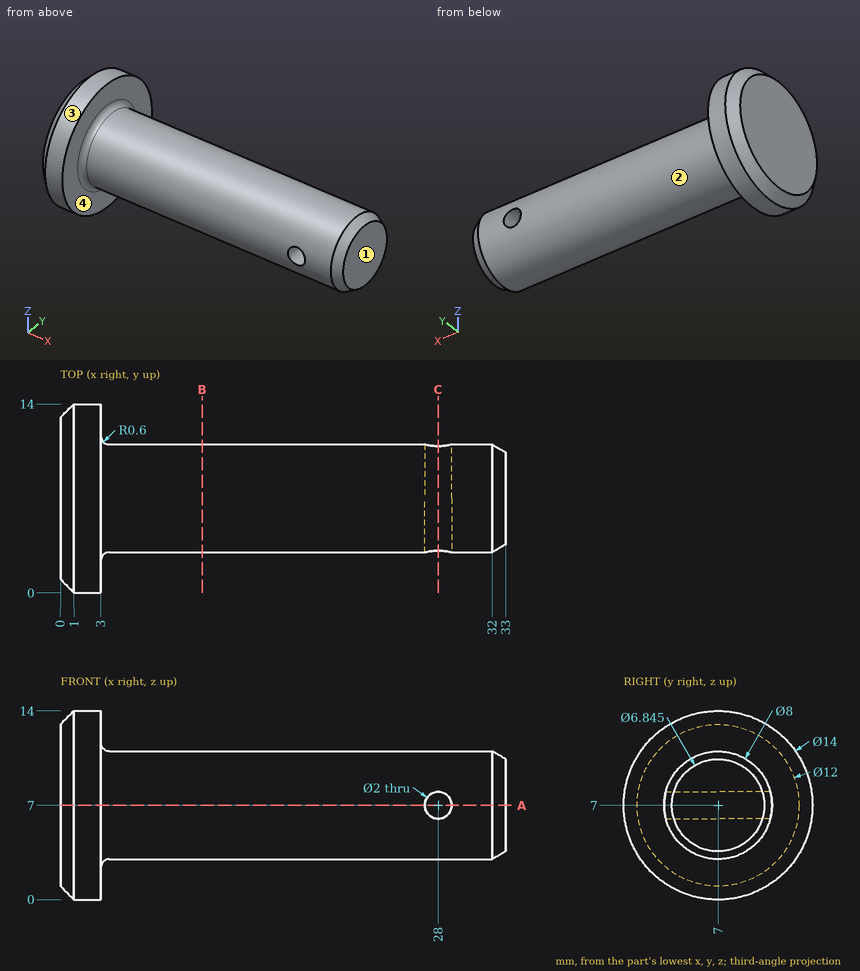
Verification items for this drawing (mm, ordinates from the low corner). A direction names the side the tool comes from. Coordinates: 2 decimals unless noted, no trailing zeros. Order: outer loops, then holes, each group sorted by start corner. A loop starts at its lowest first (then second) coordinate and runs counter-clockwise, first axis right, second up. Notation, with made-up numbers: M 82,-15.75 L 100,-15.75 A33 ccw 100,18.25 Z; hole C -37.75,54.5 d2. An arc over 180 degrees is marked long. Use CSV: the item, a comma, the result in double quotes.
Item 1: Cross-section at C-C on x = 28. Record the cut outline in (y, z).
Returned:
outline,"M 3.13,6 A4 ccw 10.87,6 Z; M 3.13,8 L 10.87,8 A4 ccw Z"
Item 2: Gauge pin test, flat ends, axial feed: pin 1 Ø4 at (x, z) = (15, 8) entering from -Y; pin 2 Ø1.5 at (y, z) = (4.5, 11.5) entering from +X (1 decimal); pin 3 Ø3 at (x, z) = (12, 4) entering from +Y. Record the tip position at first contact, or that the pin passes through.
Returned:
pin 1,"stops at y = 3"
pin 2,"stops at x = 3"
pin 3,"stops at y = 10.71"
Item 3: Mould release check, pull along Z, two halves, no side actions. Record for the marked faces 1 and 2: pulls with the +Z half, pulls with the -Z half, needs draft (parallel to the pull), parting line crosses it, or undercut.
Returned:
face 1,"needs draft"
face 2,"parting line crosses it"
Item 4: Cross-section at B-B on x = 10.5. Record the cut outline in (y, z).
Returned:
outline,"C 7,7 d8"
Item 5: Cross-section at A-A on z = 7. Record the cut outline in (x, y).
Returned:
outline,"M 0,1 L 1,0 L 3,0 L 3,2.4 A0.6 cw 3.6,3 L 27,3 L 27,11 L 3.6,11 A0.6 cw 3,11.6 L 3,14 L 1,14 L 0,13 Z; M 29,3 L 32,3 L 33,3.58 L 33,10.42 L 32,11 L 29,11 Z"
Item 6: Tool access check on the marked faces 3 and 4. Record the directions out of +Z, -Z, +X, -X, +Y, -Y that give a thin tool (end or side, any length) a straight path to the whole face; none if there is none.
Returned:
face 3,"+X, -X"
face 4,"+X"
Item 7: Thickness scan on line 1 along X through (y, z) = (9.85, 7); line 2 along X through (y, z) = (11.75, 8.75); line 3 along Z through (x, y) = (28, 6.25). Record the ranges inside material, lowest first.
Returned:
line 1,"x = 0 to 27, 29 to 33"
line 2,"x = 0 to 3"
line 3,"z = 3.07 to 6, 8 to 10.93"
